For this review, take the finished solid that the model builds, in its own axes (mm). A direction names the side the tool comes from. Give positions to 0.01 mm unless a question says otherwise; leave off trailing zeros. Order: outer loops, then holes, each group sorted by start corner. A loop starts at its lowest first (then second) coordinate and runs counter-clockwise, first axis right, second up.
from build123d import *

# Parameters (mm, degrees)
SKETCH1_W             = 50.8
SKETCH1_H             = 50.8
SKETCH1_R             = 12.7
BOSS_EXTRUDE2_DEPTH   = 31.75
BOSS_EXTRUDE5_DEPTH   = 6.35
CUT_EXTRUDE2_DEPTH    = 6.35
CUT_EXTRUDE3_DEPTH    = 6.35
SKETCH12_W            = 38.1
SKETCH12_H            = 38.1
CUT_EXTRUDE6_DEPTH    = 25.4
F_6_32_TAPPED_HOLE3_D = 2.7051
CUT_EXTRUDE7_DEPTH    = 25.4


with BuildPart() as part:
    # Sketch1 → Boss-Extrude2 (new body)
    with BuildSketch(Plane(origin=(0, 0, 0), x_dir=(1, 0, 0), z_dir=(0, 1, 0))):
        Rectangle(SKETCH1_W, SKETCH1_H)
        with Locations(Location((0, 0, 0), (0, 0, 270))):
            Circle(SKETCH1_R, mode=Mode.SUBTRACT)
    extrude(amount=BOSS_EXTRUDE2_DEPTH)

    # Sketch4 → Boss-Extrude5 (add)
    with BuildSketch(Plane(origin=(0, 0, 0), x_dir=(-1, 0, 0), z_dir=(0, -1, 0))):
        Polygon((25.4, -25.4), (-25.366380646, -25.4), (-25.366380646, -37.321328202), (37.321328153, -37.321328202), (37.321328153, -25.4), (37.321328153, 25.4), (25.4, 25.4), align=None)
    extrude(amount=-BOSS_EXTRUDE5_DEPTH)

    # Sketch11 → Cut-Extrude2 (cut)
    with BuildSketch(Plane(origin=(0, 6.35, 0), x_dir=(1, 0, 0), z_dir=(0, 1, 0))):
        with BuildLine():
            Line((-28.60675, 10.43410283), (-28.60675, 2.26589717))
            ThreePointArc((-28.60675, 2.26589717), (-30.988, -0.11535283), (-33.36925, 2.26589717))
            Line((-33.36925, 2.26589717), (-33.36925, 10.43410283))
            ThreePointArc((-33.36925, 10.43410283), (-30.988, 12.81535283), (-28.60675, 10.43410283))
        make_face()
        with BuildLine():
            Line((-29.587864683, -24.49752021), (-24.922781552, -31.202487256))
            ThreePointArc((-24.922781552, -31.202487256), (-25.517462167, -34.517160405), (-28.832135317, -33.92247979))
            Line((-28.832135317, -33.92247979), (-33.497218448, -27.217512744))
            ThreePointArc((-33.497218448, -27.217512744), (-32.902537833, -23.902839595), (-29.587864683, -24.49752021))
        make_face()
    extrude(amount=-CUT_EXTRUDE2_DEPTH, mode=Mode.SUBTRACT)

    # Sketch10 → Cut-Extrude3 (cut)
    with BuildSketch(Plane(origin=(0, 6.35, 0), x_dir=(1, 0, 0), z_dir=(0, 1, 0))):
        with BuildLine():
            Line((10.434102814, -33.36925), (2.265897186, -33.36925))
            ThreePointArc((2.265897186, -33.36925), (-0.115352814, -30.988), (2.265897186, -28.60675))
            Line((2.265897186, -28.60675), (10.434102814, -28.60675))
            ThreePointArc((10.434102814, -28.60675), (12.815352814, -30.988), (10.434102814, -33.36925))
        make_face()
    extrude(amount=-CUT_EXTRUDE3_DEPTH, mode=Mode.SUBTRACT)

    # Sketch12 → Cut-Extrude6 (cut)
    with BuildSketch(Plane(origin=(0, 0, 0), x_dir=(-1, 0, 0), z_dir=(0, -1, 0))):
        Rectangle(SKETCH12_W, SKETCH12_H)
    extrude(amount=-CUT_EXTRUDE6_DEPTH, mode=Mode.SUBTRACT)

    # #6-32 Tapped Hole3 (through all)
    with Locations(Plane(origin=(7.158073922, 31.75, 16.96706293), x_dir=(0, 0, 1), z_dir=(0, 1, 0))):
        with Locations((0, 0), (-25.125718539, -23.79160959)):
            Hole(F_6_32_TAPPED_HOLE3_D / 2)

    # Sketch18 → Cut-Extrude7 (cut)
    with BuildSketch(Plane(origin=(0, 0, -25.4), x_dir=(-1, 0, 0), z_dir=(0, 0, -1))):
        with BuildLine():
            Line((4.620408953, 25.334287556), (4.620408953, 9.209712444))
            ThreePointArc((4.620408953, 9.209712444), (0, 4.589303492), (-4.620408953, 9.209712444))
            Line((-4.620408953, 9.209712444), (-4.620408953, 25.334287556))
            ThreePointArc((-4.620408953, 25.334287556), (0, 29.954696508), (4.620408953, 25.334287556))
        make_face()
    extrude(amount=-CUT_EXTRUDE7_DEPTH, mode=Mode.SUBTRACT)


solid = part.part
1) We need section D-D on z = -21. Give the boundary of the cut face in (x, y), then the cut area to 3 significant figures.
Answer sheet:
outline: (-37.32, 0) - (25.4, 0) - (25.4, 31.75) - (-25.4, 31.75) - (-25.4, 6.35) - (-37.32, 6.35) - close; hole (-4.62, 9.21) arc R4.62 ccw to (4.62, 9.21) - (4.62, 25.33) arc R4.62 ccw to (-4.62, 25.33) - close
area: 1,470 mm2
2) Clearance check with flat-ended pins moving along their axes: pin 1 (1 mm diameter, centred on x = -6, y = 20, fed in from +Z); pin 2 (3 mm diameter, centred on y = 2.5, z = 28.5, fed in from +X); pin 3 (5 mm diameter, centred on y = 19, z = -22, fed in from -X); pin 4 (1.6 mm diameter, centred on x = -16.63, z = -8.16, fed in from +Y). State where each tip first meets the part, or that it passes through.
Answer sheet:
pin 1: stops at z = 25.4
pin 2: stops at x = 25.37
pin 3: stops at x = -25.4
pin 4: passes through
3) We need section A-A on z = 6.5. Give the boundary of the cut face in (x, y), then the cut area to 3 significant figures.
Answer sheet:
outline: (-37.32, 0) - (-19.05, 0) - (-19.05, 25.4) - (-10.91, 25.4) - (-10.91, 31.75) - (-25.4, 31.75) - (-25.4, 6.35) - (-37.32, 6.35) - close; (10.91, 25.4) - (19.05, 25.4) - (19.05, 0) - (25.4, 0) - (25.4, 31.75) - (10.91, 31.75) - close
area: 582 mm2
4) Tool access review of faces 1 (the face through (-25.4, 19, 0)), 2 (the face through (-19.05, 13, 0)), 3 (the face through (-0.115, 3.219, 31.04)): name each direction out of +Z, -Z, +X, -X, +Y, -Y from which nothing blocks a thin tool from reaching the whole face with its end or side.
Answer sheet:
face 1: +Z, -Z, -X, +Y
face 2: -Y
face 3: +Y, -Y
5) Draft analysis for pull direction Y (two halves, no side actions). For faces 4 (the face through (5, 25.4, 12)), 5 (the face through (19.05, 13, 0)), 6 (the face through (-4.62, 17, -22)), 7 (the face through (4.62, 17, -22)), state which applies: +Y half, -Y half, draft (parallel to the pull), parting line (faces both ways), or undercut.
Answer sheet:
face 4: -Y half
face 5: draft
face 6: undercut
face 7: undercut
6) We need section C-C on y = 16. Give the boundary of the cut face in (x, z).
Answer sheet:
outline: (-25.4, -25.4) - (-4.62, -25.4) - (-4.62, -19.05) - (-19.05, -19.05) - (-19.05, 19.05) - (19.05, 19.05) - (19.05, -19.05) - (4.62, -19.05) - (4.62, -25.4) - (25.4, -25.4) - (25.4, 25.4) - (-25.4, 25.4) - close
7) To check wall thickness, follow line 1 (X direction, y = 18.5, z = -13); line 2 (X direction, y = 29.25, z = 0). State the ranges of each line that lie inside material, in increasing order.
Answer sheet:
line 1: x = -25.4 to -19.05, 19.05 to 25.4
line 2: x = -25.4 to -12.7, 12.7 to 25.4
8) We need section B-B on x = -31. Give the boundary of the cut face in (y, z), then the cut area to 3 significant figures.
Answer sheet:
outline: (0, -25.4) - (6.35, -25.4) - (6.35, -12.82) - (0, -12.82) - close; (0, 0.12) - (6.35, 0.12) - (6.35, 23.54) - (0, 23.54) - close; (0, 30.81) - (6.35, 30.81) - (6.35, 37.32) - (0, 37.32) - close
area: 270 mm2
